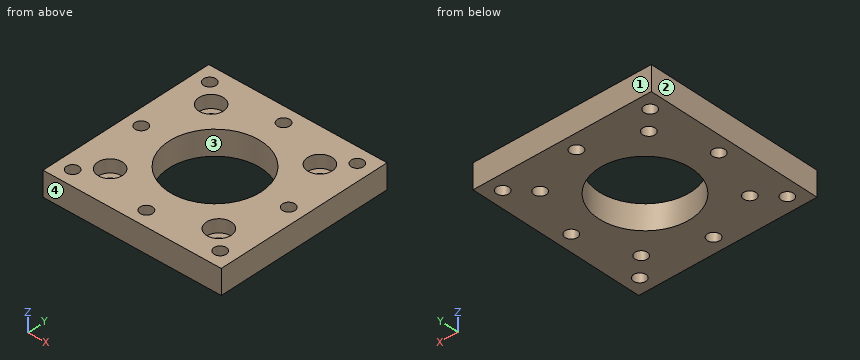
```python
from build123d import *

# Parameters (mm, degrees)
SKETCH1_W           = 58
SKETCH1_H           = 58
SKETCH1_R           = 15
SKETCH1_R_2         = 2
BOSS_EXTRUDE1_DEPTH = 8
SKETCH3_R           = 2
CUT_EXTRUDE1_DEPTH  = 42.785164832
SKETCH4_R           = 4
CUT_EXTRUDE2_DEPTH  = 4.2


with BuildPart() as part:
    # Sketch1 → Boss-Extrude1 (new body)
    with BuildSketch(Plane.XY):
        Rectangle(SKETCH1_W, SKETCH1_H)
        Circle(SKETCH1_R, mode=Mode.SUBTRACT)
        with Locations((0, 24)):
            Circle(SKETCH1_R_2, mode=Mode.SUBTRACT)
        with Locations((-24, 24)):
            Circle(SKETCH1_R_2, mode=Mode.SUBTRACT)
        with Locations((24, 0)):
            Circle(SKETCH1_R_2, mode=Mode.SUBTRACT)
        with Locations((0, -24)):
            Circle(SKETCH1_R_2, mode=Mode.SUBTRACT)
        with Locations((-24, 0)):
            Circle(SKETCH1_R_2, mode=Mode.SUBTRACT)
        with Locations(Location((24, -24, 0), (0, 0, 180))):
            Circle(SKETCH1_R_2, mode=Mode.SUBTRACT)
        with Locations((24, 24)):
            Circle(SKETCH1_R_2, mode=Mode.SUBTRACT)
        with Locations(Location((-24, -24, 0), (0, 0, 180))):
            Circle(SKETCH1_R_2, mode=Mode.SUBTRACT)
    extrude(amount=BOSS_EXTRUDE1_DEPTH)

    # Sketch3 → Cut-Extrude1 (cut, through all)
    with BuildSketch(Plane(origin=(0, 0, 0), x_dir=(-1, 0, 0), z_dir=(0, 0, -1))):
        with Locations((-17.673408237, 17.681929795)):
            Circle(SKETCH3_R)
        with Locations((17.681929795, 17.673408237)):
            Circle(SKETCH3_R)
        with Locations((17.673408237, -17.681929795)):
            Circle(SKETCH3_R)
        with Locations((-17.681929795, -17.673408237)):
            Circle(SKETCH3_R)
    extrude(amount=-CUT_EXTRUDE1_DEPTH, mode=Mode.SUBTRACT)

    # Sketch4 → Cut-Extrude2 (cut)
    with BuildSketch(Plane.XY.offset(8)):
        with Locations((-17.681929795, 17.673408237)):
            Circle(SKETCH4_R)
        with Locations((17.673408237, 17.681929795)):
            Circle(SKETCH4_R)
        with Locations((17.681929795, -17.673408237)):
            Circle(SKETCH4_R)
        with Locations((-17.673408237, -17.681929795)):
            Circle(SKETCH4_R)
    extrude(amount=-CUT_EXTRUDE2_DEPTH, mode=Mode.SUBTRACT)


solid = part.part
```
Geometry: final body of the model. Coordinates: model frame, mm. Face numbers are marked on the shaded views. Round coordinates to 2 decimals unless told otherwise and drop trailing zeros. Write each loop counter-clockwise with the first axis right and the second up, starting at its lowest first coordinate (ties: lowest second). Pieces come first, ordered by that corner, then holes. Notation, with made-up numbers: (78, 89) -> (89, 89) arc R15 ccw to (89, 96) -> close; hole circle Ø1 at (11, 81.5). An arc over 180 degrees is marked (long way). Return JSON: item names as keys, results as strings.
Q1. Section D-D on y = 10. Return the cut outline in (x, z).
From the geometry:
{"outline": "(-29, 0) -> (-11.18, 0) -> (-11.18, 8) -> (-29, 8) -> close; (11.18, 0) -> (29, 0) -> (29, 8) -> (11.18, 8) -> close"}
Q2. Section C-C on x = -9. Return the cut outline in (y, z).
From the geometry:
{"outline": "(-29, 0) -> (-12, 0) -> (-12, 8) -> (-29, 8) -> close; (12, 0) -> (29, 0) -> (29, 8) -> (12, 8) -> close"}
Q3. First-contact query: pin 1 Ø4.5 at (x, y) = (24, 0) entering from -Z; pin 2 Ø2.5 at (x, y) = (-24, -24) entering from +Z; pin 3 Ø7 at (x, y) = (17.67, 17.68) entering from +Z. Flat tips, straight axial feed; report the tip coordinate or a pass-through.
From the geometry:
{"pin 1": "z = 0", "pin 2": "through", "pin 3": "z = 3.8"}
Q4. Section A-A on x = -24. Return the cut outline in (y, z), and give its area (3 significant figures).
From the geometry:
{"outline": "(-29, 0) -> (-26, 0) -> (-26, 8) -> (-29, 8) -> close; (-22, 0) -> (-2, 0) -> (-2, 8) -> (-22, 8) -> close; (2, 0) -> (22, 0) -> (22, 8) -> (2, 8) -> close; (26, 0) -> (29, 0) -> (29, 8) -> (26, 8) -> close", "area": "368 mm2"}
Q5. Mould query, pull axis Y, two halves, no side actions, for the marked faces 1, 2, 3 and 4. Classes: +Y half, -Y half, draft (parallel to the pull), parting line (faces both ways), or undercut.
From the geometry:
{"face 1": "+Y half", "face 2": "draft", "face 3": "undercut", "face 4": "-Y half"}
Q6. Ray query, line 1 (X direction, y = 18, z = 7); line 2 (Y direction, x = -24, z = 2); line 3 (Y direction, x = 0, z = 5.25). Return the intervals inside material, ascending.
From the geometry:
{"line 1": "-29 to -21.67, -13.7 to 13.69, 21.66 to 29", "line 2": "-29 to -26, -22 to -2, 2 to 22, 26 to 29", "line 3": "-29 to -26, -22 to -15, 15 to 22, 26 to 29"}
Q7. Section B-B on y = 0. Return the cut outline in (x, z).
From the geometry:
{"outline": "(-29, 0) -> (-26, 0) -> (-26, 8) -> (-29, 8) -> close; (-22, 0) -> (-15, 0) -> (-15, 8) -> (-22, 8) -> close; (15, 0) -> (22, 0) -> (22, 8) -> (15, 8) -> close; (26, 0) -> (29, 0) -> (29, 8) -> (26, 8) -> close"}
